Design review of the part shown in the three views and the two pictorial views. Dimensions are in mm from the part's minimum x, y and z. A direction names the side the tool comes from. Round coordinates to 2 decimals unless told otherwise and drop trailing zeros. Order: outer loops, then holes, each group sorted by start corner. A loop starts at its lowest first (then second) coordinate and runs counter-clockwise, first axis right, second up.
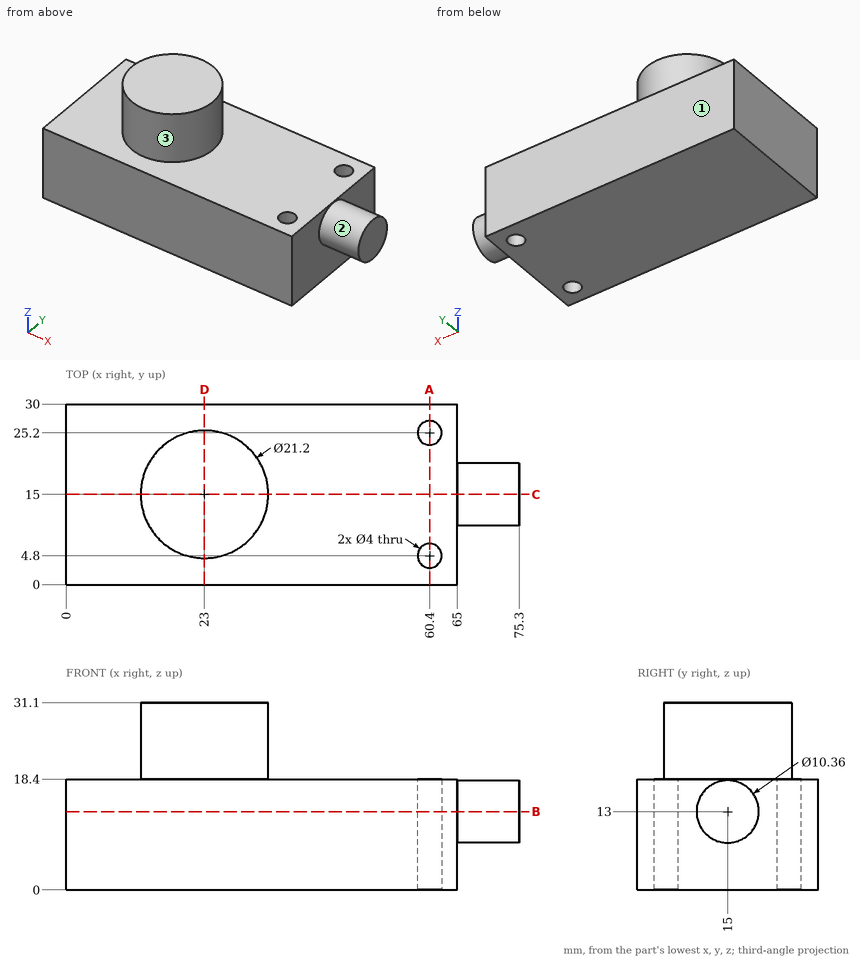
1) For the marked faces 1, 2 and 3, list the 3-axis set-ups (+Z, -Z, +X, -X, +Y, -Y) from which the entire face can be reached by the end or side of a thin tool; tool diameter is ignored.
Results:
face 1: +Z, -Z, +X, -X, +Y
face 2: +X
face 3: +Z
2) Take a section at B-B on z = 13. Give the boundary of the cut face in (x, y).
Results:
outline: (0, 0) - (65, 0) - (65, 9.82) - (75.3, 9.82) - (75.3, 20.18) - (65, 20.18) - (65, 30) - (0, 30) - close; hole circle Ø4 at (60.4, 4.8); hole circle Ø4 at (60.4, 25.2)
3) To check wall thickness, follow line 1 along Y through (x, z) = (60.4, 7.75); line 2 along Z through (x, y) = (50.5, 12.25); line 3 along X through (y, z) = (10, 16). State the ranges of each line that lie inside material, in increasing order.
Results:
line 1: y = 0 to 2.8, 6.8 to 23.2, 27.2 to 30
line 2: z = 0 to 18.4
line 3: x = 0 to 65
4) Take a section at A-A on x = 60.4. Give the boundary of the cut face in (y, z).
Results:
outline: (0, 0) - (2.8, 0) - (2.8, 18.4) - (0, 18.4) - close; (6.8, 0) - (23.2, 0) - (23.2, 18.4) - (6.8, 18.4) - close; (27.2, 0) - (30, 0) - (30, 18.4) - (27.2, 18.4) - close
5) Take a section at D-D on x = 23. Give the boundary of the cut face in (y, z).
Results:
outline: (0, 0) - (30, 0) - (30, 18.4) - (25.6, 18.4) - (25.6, 31.1) - (4.4, 31.1) - (4.4, 18.4) - (0, 18.4) - close
6) Clearance check with flat-ended pins moving along their axes: P1, Ø5.5, axis at y = 8.5, z = 10.5, coming from the +X side; P2, Ø5, axis at x = 60.4, y = 25.2, coming from the +Z side; P3, Ø1.5, axis at x = 67.5, y = 12.5, coming from the -Z side. State where each tip first meets the part, or that it passes through.
Results:
P1: stops at x = 75.3
P2: stops at z = 18.4
P3: stops at z = 8.12
7) Take a section at C-C on y = 15. Give the boundary of the cut face in (x, z), plus the area to 3 significant figures.
Results:
outline: (0, 0) - (65, 0) - (65, 7.82) - (75.3, 7.82) - (75.3, 18.18) - (65, 18.18) - (65, 18.4) - (33.6, 18.4) - (33.6, 31.1) - (12.4, 31.1) - (12.4, 18.4) - (0, 18.4) - close
area: 1,570 mm2
